```python
from build123d import *

# Parameters (mm, degrees)
SKETCH1_R           = 1.8161
BOSS_EXTRUDE1_DEPTH = 38.1
CHAMFER1_SIZE       = 3.175
CHAMFER1_SIZE2      = 1.155605494
BOSS_EXTRUDE2_START = 2.54
SKETCH2_R           = 1.8161
BOSS_EXTRUDE2_DEPTH = 2.54
BOSS_EXTRUDE3_START = 17.78
SKETCH3_R           = 1.8161
BOSS_EXTRUDE3_DEPTH = 17.78
BOSS_EXTRUDE4_DEPTH = 7.62
BOSS_EXTRUDE5_START = 6.35
BOSS_EXTRUDE5_DEPTH = 6.35
BOSS_EXTRUDE6_DEPTH = 241.3
FILLET2_R           = 0.762


with BuildPart() as part:
    # Sketch1 → Boss-Extrude1 (new body)
    with BuildSketch(Plane.XY):
        with Locations(Location((0, 0, 0), (0, 0, 180))):
            Circle(SKETCH1_R)
    extrude(amount=BOSS_EXTRUDE1_DEPTH)

    # Chamfer1
    chamfer1_edges = [part.edges().sort_by_distance(p)[0] for p in [
        (1.8161, 0, 38.1),
    ]]
    chamfer1_side = [part.faces().sort_by_distance(p)[0] for p in [
        (1.8161, 0, 19.05),
    ]]
    chamfer(chamfer1_edges, length=CHAMFER1_SIZE, length2=CHAMFER1_SIZE2, reference=chamfer1_side[0])

    # Sketch2 → Boss-Extrude2 (add)
    with BuildSketch(Plane(origin=(0, 0, 0), x_dir=(-1, 0, 0), z_dir=(0, 0, -1)).offset(BOSS_EXTRUDE2_START)):
        Circle(SKETCH2_R)
    extrude(amount=-BOSS_EXTRUDE2_DEPTH)

    # Sketch3 → Boss-Extrude3 (add)
    with BuildSketch(Plane(origin=(0, 0, -2.54), x_dir=(-1, 0, 0), z_dir=(0, 0, -1)).offset(BOSS_EXTRUDE3_START)):
        Circle(SKETCH3_R)
    extrude(amount=-BOSS_EXTRUDE3_DEPTH)

    # Sketch4 → Boss-Extrude4 (add)
    with BuildSketch(Plane(origin=(0, 0, -20.32), x_dir=(-1, 0, 0), z_dir=(0, 0, -1))):
        with BuildLine():
            Line((-1.524, 1.016), (1.524, 1.016))
            ThreePointArc((1.524, 1.016), (2.54, 0), (1.524, -1.016))
            Line((1.524, -1.016), (-1.524, -1.016))
            ThreePointArc((-1.524, -1.016), (-2.54, 0), (-1.524, 1.016))
        make_face()
    extrude(amount=BOSS_EXTRUDE4_DEPTH)

    # Sketch5 → Boss-Extrude5 (add)
    with BuildSketch(Plane(origin=(0, 0, -27.94), x_dir=(-1, 0, 0), z_dir=(0, 0, -1)).offset(BOSS_EXTRUDE5_START)):
        with BuildLine():
            ThreePointArc((-1.50542625, -1.01583021), (0, -1.8161), (1.50542625, -1.01583021))
            ThreePointArc((1.50542625, -1.01583021), (0, 1.8161), (-1.50542625, -1.01583021))
        make_face()
    extrude(amount=-BOSS_EXTRUDE5_DEPTH)

    # Sketch6 → Boss-Extrude6 (add)
    with BuildSketch(Plane(origin=(0, 0, -34.29), x_dir=(-1, 0, 0), z_dir=(0, 0, -1))):
        with BuildLine():
            Line((0.6985, -0.6985), (-0.6985, -0.6985))
            ThreePointArc((-0.6985, -0.6985), (-1.397, 0), (-0.6985, 0.6985))
            Line((-0.6985, 0.6985), (0.6985, 0.6985))
            ThreePointArc((0.6985, 0.6985), (1.397, 0), (0.6985, -0.6985))
        make_face()
    extrude(amount=BOSS_EXTRUDE6_DEPTH)

    # Fillet2
    # the kernel refuses this fillet: 0.762 mm, written as the material it adds along each edge
    with BuildSketch(Plane(origin=(-3.410311665, -1.016, -20.32), x_dir=(0, -1, 0), z_dir=(1, 0, 0))) as fillet2_piece_1_section:
        with BuildLine():
            CenterArc((FILLET2_R, FILLET2_R), FILLET2_R, 180, 90)
            Line((0, FILLET2_R), (0, 0))
            Line((0, 0), (FILLET2_R, 0))
        make_face()
    fillet2_piece_1 = extrude(amount=6.820623331, mode=Mode.PRIVATE)
    fillet2_piece_1 = fillet2_piece_1 & Plane(origin=(0, 0, -20.517592364), x_dir=(-1, 0, 0), z_dir=(0, 0, -1)) * Cylinder(1.8161, 17, mode=Mode.PRIVATE)
    add(fillet2_piece_1)
    with BuildSketch(Plane(origin=(3.410311665, 1.016, -20.32), x_dir=(0, 1, 0), z_dir=(-1, 0, 0))) as fillet2_piece_2_section:
        with BuildLine():
            CenterArc((FILLET2_R, FILLET2_R), FILLET2_R, 180, 90)
            Line((0, FILLET2_R), (0, 0))
            Line((0, 0), (FILLET2_R, 0))
        make_face()
    fillet2_piece_2 = extrude(amount=6.820623331, mode=Mode.PRIVATE)
    fillet2_piece_2 = fillet2_piece_2 & Plane(origin=(0, 0, -20.517592364), x_dir=(-1, 0, 0), z_dir=(0, 0, -1)) * Cylinder(1.8161, 17, mode=Mode.PRIVATE)
    add(fillet2_piece_2)
    with BuildSketch(Plane(origin=(-3.410311665, -1.016, -27.94), x_dir=(0, 0, 1), z_dir=(1, 0, 0))) as fillet2_piece_3_section:
        with BuildLine():
            CenterArc((FILLET2_R, FILLET2_R), FILLET2_R, 180, 90)
            Line((0, FILLET2_R), (0, 0))
            Line((0, 0), (FILLET2_R, 0))
        make_face()
    fillet2_piece_3 = extrude(amount=6.820623331, mode=Mode.PRIVATE)
    fillet2_piece_3 = fillet2_piece_3 & Plane(origin=(0, 0, -27.742407671), x_dir=(0.8289335664335663, -0.5593470679638254, 0), z_dir=(0, 0, -1)) * Cylinder(1.8161, 17, mode=Mode.PRIVATE)
    add(fillet2_piece_3)
    with BuildSketch(Plane(origin=(3.410311665, 1.016, -27.94), x_dir=(0, 0, 1), z_dir=(-1, 0, 0))) as fillet2_piece_4_section:
        with BuildLine():
            CenterArc((FILLET2_R, FILLET2_R), FILLET2_R, 180, 90)
            Line((0, FILLET2_R), (0, 0))
            Line((0, 0), (FILLET2_R, 0))
        make_face()
    fillet2_piece_4 = extrude(amount=6.820623331, mode=Mode.PRIVATE)
    fillet2_piece_4 = fillet2_piece_4 & Plane(origin=(0, 0, -27.742407638), x_dir=(0.8289335664335663, -0.5593470679638254, 0), z_dir=(0, 0, -1)) * Cylinder(1.8161, 17, mode=Mode.PRIVATE)
    add(fillet2_piece_4)


solid = part.part
```
Part model, mm, in its own coordinate system. Round coordinates to 2 decimals unless told otherwise and drop trailing zeros. Write each loop counter-clockwise with the first axis right and the second up, starting at its lowest first coordinate (ties: lowest second). Pieces come first, ordered by that corner, then holes. Notation, with made-up numbers: M 71,29.5 L 97,29.5 A18 cw 97,36.5 Z; hole C 85.25,40.5 d5. An arc over 180 degrees is marked long. Answer as CSV lines item,"result". Start each with the question number.
1) Band-saw the part on A-A (y = 0). List the corners of the cut face in (x, z) (1 decimal), then the cut area to 3 significant figures.
2) Band-saw the part on B-B (z = -216). List the corners of the cut face in (x, y), then the cut area to 3 significant figures.
3) Drill centre lines: L1, parallel to X at y = 0.05, z = 19; L2, parallel to Z at x = 2.2, y = -0.3; L3, parallel to Y at x = 1.25, z = -63.5. Where is each one in solid material? Low to high.
4) Drop flat-ended pins along their axis: pin 1 (1.5 mm diameter, centred on y = 1, z = -31, fed in from -X); pin 2 (1.5 mm diameter, centred on x = 0.5, z = -176, fed in from -Y); pin 3 (0.8 mm diameter, centred on x = -2, y = -0.5, fed in from -Z). Give the stop position or say it passes through.
Worked out:
1,outline,"M -2.5,-27.9 L -1.8,-27.9 L -1.8,-34.3 L -1.4,-34.3 L -1.4,-275.6 L 1.4,-275.6 L 1.4,-34.3 L 1.8,-34.3 L 1.8,-27.9 L 2.5,-27.9 L 2.5,-20.3 L 1.8,-20.3 L 1.8,34.9 L 0.7,38.1 L -0.7,38.1 L -1.8,34.9 L -1.8,-20.3 L -2.5,-20.3 Z"
1,area,"944 mm²"
2,outline,"M -0.7,-0.7 L 0.7,-0.7 A0.7 ccw 0.7,0.7 L -0.7,0.7 A0.7 ccw Z"
2,area,"3.48 mm²"
3,L1,"-1.82 to 1.82"
3,L2,"-27.94 to -20.32"
3,L3,"-0.43 to 0.43"
4,pin 1,"x = -1.8"
4,pin 2,"y = -0.7"
4,pin 3,"z = -34.29"
